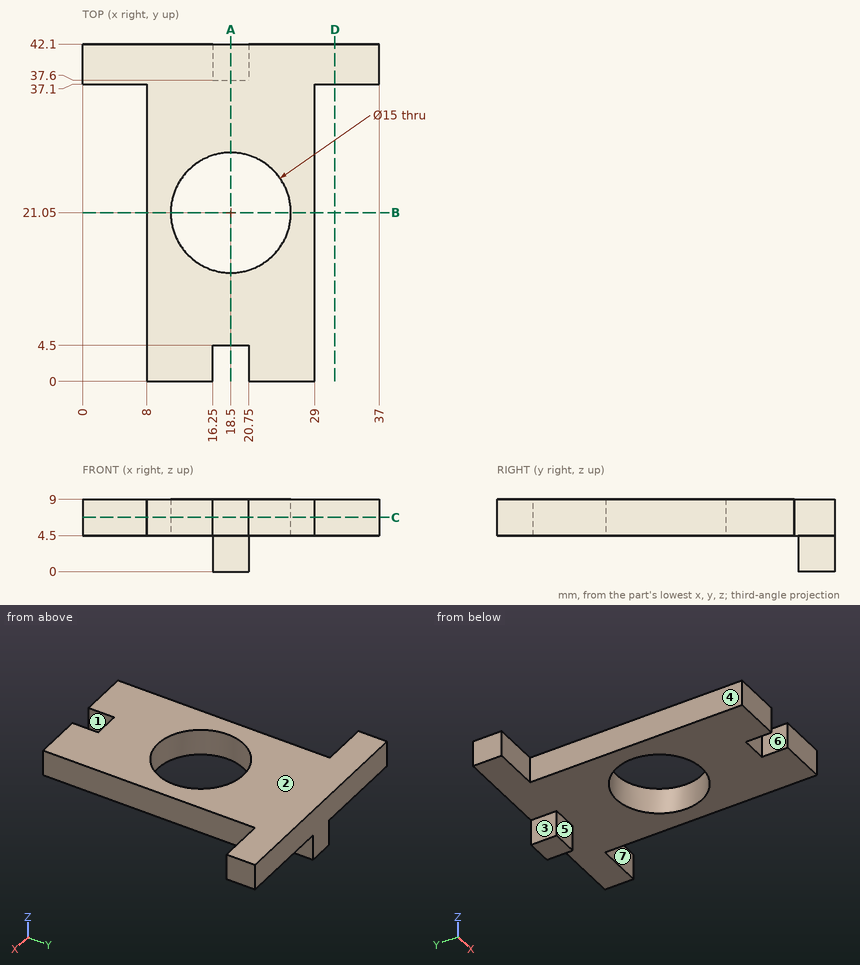
Part print with two shaded views. Sizes in mm from the minimum x, y, z corner. A direction names the side the tool comes from. Coordinates: 2 decimals unless noted, no trailing zeros. Write each loop counter-clockwise with the first axis right and the second up, starting at its lowest first coordinate (ties: lowest second). Pieces come first, ordered by that corner, then holes. Notation, with made-up numbers: (-18.5, 24.5) - (-11.5, 24.5) arc R8 cw to (-11.5, 30.5) - close; hole circle Ø1 at (3.5, 12.5). An arc over 180 degrees is marked (long way). Use a Markdown table: item, result. Add a question column.
Item 1: Band-saw the part on B-B, the plane y = 21.05. Write the cut outline in (x, z).
Item 2: Drill centre lines: line 1 along Y through (x, z) = (18.5, 8); line 2 along X through (y, z) = (30.5, 8.5); line 3 along Z through (x, y) = (27.5, 38.5). Where is each one in solid material? Low to high.
Item 3: Drop flat-ended pins along their axis: pin 1 (3.5 mm diameter, centred on y = 14, z = 7, fed in from +X); pin 2 (5 mm diameter, centred on y = 18.5, z = 8, fed in from -X); pin 3 (5 mm diameter, centred on y = 40, z = 1, fed in from -X); pin 4 (6 mm diameter, centred on x = 6, y = 28, fed in from +Z). Give the stop position or say it passes through.
Item 4: 3-axis set-ups, long thin cutter, end or side, ignore diameter. For the marked faces 4, 5, 6 and 7: which of +Z, -Z, +X, -X, +Y, -Y reach the whole face in a straight line?
Item 5: Two-plate mould, pull along X, no slides. Class the marked faces 1, 2 and 3: pulls with the +X half, pulls with the -X half, needs draft (parallel to the pull), parting line crosses it, or undercut.
Item 6: Band-saw the part on D-D, the plane x = 31.5. Write the cut outline in (y, z).
Item 7: Band-saw the part on A-A, the plane x = 18.5. Write the cut outline in (y, z), and give its area (3 significant figures).
Item 8: Band-saw the part on C-C, the plane z = 6.75. Write the cut outline in (x, y).
A:
| question | item | result |
|---|---|---|
| 1 | outline | (8, 4.5) - (11, 4.5) - (11, 9) - (8, 9) - close; (26, 4.5) - (29, 4.5) - (29, 9) - (26, 9) - close |
| 2 | line 1 | y = 4.5 to 13.55, 28.55 to 42.1 |
| 2 | line 2 | x = 8 to 29 |
| 2 | line 3 | z = 4.5 to 9 |
| 3 | pin 1 | stops at x = 29 |
| 3 | pin 2 | stops at x = 8 |
| 3 | pin 3 | stops at x = 16.25 |
| 3 | pin 4 | stops at z = 9 |
| 4 | face 4 | +Z, -Z, -X, -Y |
| 4 | face 5 | -Z, +X, -X, -Y |
| 4 | face 6 | +Z, -Z, -Y |
| 4 | face 7 | +Z, -Z, +X, -Y |
| 5 | face 1 | undercut |
| 5 | face 2 | needs draft |
| 5 | face 3 | pulls with the -X half |
| 6 | outline | (37.1, 4.5) - (42.1, 4.5) - (42.1, 9) - (37.1, 9) - close |
| 7 | outline | (4.5, 4.5) - (13.55, 4.5) - (13.55, 9) - (4.5, 9) - close; (28.55, 4.5) - (37.6, 4.5) - (37.6, 0) - (42.1, 0) - (42.1, 9) - (28.55, 9) - close |
| 7 | area | 122 mm² |
| 8 | outline | (0, 37.1) - (8, 37.1) - (8, 0) - (16.25, 0) - (16.25, 4.5) - (20.75, 4.5) - (20.75, 0) - (29, 0) - (29, 37.1) - (37, 37.1) - (37, 42.1) - (0, 42.1) - close; hole circle Ø15 at (18.5, 21.05) |
